The figure shows three views and two pictorial views of one solid part (mm, origin at its lowest corner). Answer the questions. A direction names the side the tool comes from. Coordinates: 2 decimals unless noted, no trailing zeros. Write each loop counter-clockwise with the first axis right and the second up, starting at its lowest first coordinate (ties: lowest second). Pieces come first, ordered by that corner, then holes.
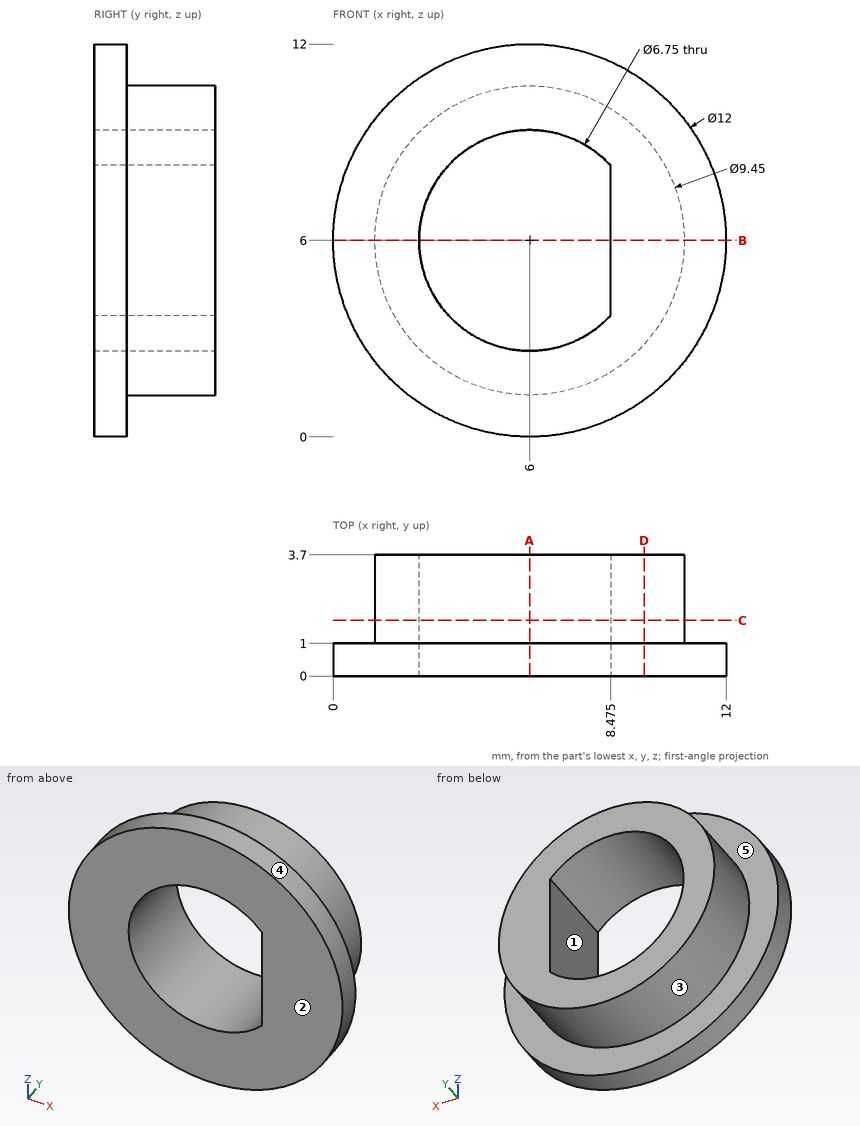
1. Find the intervals of material crossed by L1, parallel to X at y = 1.85, z = 6 (3 decimals); L2, parallel to Y at x = 9.25, z = 10.25; L3, parallel to X at y = 0.5, z = 4 (3 decimals), in increasing order.
Results found:
L1: x = 1.275 to 2.625, 8.475 to 10.725
L2: y = 0 to 1
L3: x = 0.343 to 3.281, 8.475 to 11.657
2. Section C-C on y = 1.7 is taken. Give the vertices of the cut face in (x, z) (3 decimals), then the cut area to 3 significant figures.
Results found:
outline: circle Ø9.45 at (6, 6); hole (8.475, 3.705) - (8.475, 8.295) arc R3.375 ccw (long way) to start
area: 37.2 mm2
3. A tool of negligible diameter and unlimited length cuts with its end or side. For the marked faces 4 and 5, from which of +Z, -Z, +X, -X, +Y, -Y can it reach the whole face along a straight path? Write none if from no direction.
Results found:
face 4: +Y, -Y
face 5: +Y
4. A flat-ended cylindrical pin translates along its axis: P1, Ø4, axis at x = 6, z = 6, coming from the +Y side. Find the tip coordinate at first contact, or state that the pin passes through.
Results found:
P1: passes through
5. Section D-D on x = 9.5 is taken. Give the vertices of the cut face in (y, z), then the cut area to 3 significant figures.
Results found:
outline: (0, 1.13) - (1, 1.13) - (1, 2.83) - (3.7, 2.83) - (3.7, 9.17) - (1, 9.17) - (1, 10.87) - (0, 10.87) - close
area: 26.9 mm2
6. Section B-B on z = 6 is taken. Give the vertices of the cut face in (x, y) (3 decimals), then the cut area to 3 significant figures.
Results found:
outline: (0, 0) - (2.625, 0) - (2.625, 3.7) - (1.275, 3.7) - (1.275, 1) - (0, 1) - close; (8.475, 0) - (12, 0) - (12, 1) - (10.725, 1) - (10.725, 3.7) - (8.475, 3.7) - close
area: 15.9 mm2
7. Section A-A on x = 6 is taken. Give the vertices of the cut face in (y, z) (3 decimals), then the cut area to 3 significant figures.
Results found:
outline: (0, 0) - (1, 0) - (1, 1.275) - (3.7, 1.275) - (3.7, 2.625) - (0, 2.625) - close; (0, 9.375) - (3.7, 9.375) - (3.7, 10.725) - (1, 10.725) - (1, 12) - (0, 12) - close
area: 12.5 mm2
8. For a pull along X with two mould halves and no side action, classify the marked faces 1, 2 and 3 as pulls with the +X half, pulls with the -X half, needs draft (parallel to the pull), parting line crosses it, or undercut.
Results found:
face 1: undercut
face 2: needs draft
face 3: parting line crosses it
